```python
from build123d import *

# Parameters (mm, degrees)
ESQUISSE1_R              = 50
BOSS_EXTRU_1_DEPTH       = 22
ESQUISSE5_R              = 6
ENL_V_MAT_EXTRU_6_DEPTH  = 22
ESQUISSE7_R              = 6
ENL_V_MAT_EXTRU_7_DEPTH  = 22
ESQUISSE8_R              = 6
ENL_V_MAT_EXTRU_8_DEPTH  = 22
ESQUISSE9_R              = 6
ENL_V_MAT_EXTRU_9_DEPTH  = 22
ESQUISSE10_R             = 6
ENL_V_MAT_EXTRU_10_DEPTH = 22
ESQUISSE11_R             = 6
ENL_V_MAT_EXTRU_11_DEPTH = 22
ESQUISSE12_R             = 6
ENL_V_MAT_EXTRU_12_DEPTH = 22
ESQUISSE13_R             = 6
ENL_V_MAT_EXTRU_13_DEPTH = 22
ESQUISSE14_R             = 10
ENL_V_MAT_EXTRU_15_DEPTH = 18
ESQUISSE15_R             = 2
ENL_V_MAT_EXTRU_16_DEPTH = 4


with BuildPart() as part:
    # Esquisse1 → Boss.-Extru.1 (new body)
    with BuildSketch(Plane(origin=(0, 0, 0), x_dir=(1, 0, 0), z_dir=(0, 1, 0))):
        with Locations(Location((0, 0, 0), (0, 0, 270))):
            Circle(ESQUISSE1_R)
    extrude(amount=BOSS_EXTRU_1_DEPTH)

    # Esquisse5 → Enlèv. mat.-Extru.6 (cut)
    with BuildSketch(Plane(origin=(0, 0, 0), x_dir=(-1, 0, 0), z_dir=(0, -1, 0))):
        with Locations(Location((-17.68, 17.68, 0), (0, 0, 90))):
            Circle(ESQUISSE5_R)
    extrude(amount=-ENL_V_MAT_EXTRU_6_DEPTH, mode=Mode.SUBTRACT)

    # Esquisse7 → Enlèv. mat.-Extru.7 (cut)
    with BuildSketch(Plane(origin=(0, 0, 0), x_dir=(-1, 0, 0), z_dir=(0, -1, 0))):
        with Locations(Location((18.058126749, -17.68, 0), (0, 0, 90))):
            Circle(ESQUISSE7_R)
    extrude(amount=-ENL_V_MAT_EXTRU_7_DEPTH, mode=Mode.SUBTRACT)

    # Esquisse8 → Enlèv. mat.-Extru.8 (cut)
    with BuildSketch(Plane(origin=(0, 0, 0), x_dir=(-1, 0, 0), z_dir=(0, -1, 0))):
        with Locations(Location((17.68, 17.68, 0), (0, 0, 90))):
            Circle(ESQUISSE8_R)
    extrude(amount=-ENL_V_MAT_EXTRU_8_DEPTH, mode=Mode.SUBTRACT)

    # Esquisse9 → Enlèv. mat.-Extru.9 (cut)
    with BuildSketch(Plane(origin=(0, 0, 0), x_dir=(-1, 0, 0), z_dir=(0, -1, 0))):
        with Locations(Location((-17.68, -17.68, 0), (0, 0, 90))):
            Circle(ESQUISSE9_R)
    extrude(amount=-ENL_V_MAT_EXTRU_9_DEPTH, mode=Mode.SUBTRACT)

    # Esquisse10 → Enlèv. mat.-Extru.10 (cut)
    with BuildSketch(Plane.XZ):
        with Locations(Location((0, 25, 0), (0, 0, 270))):
            Circle(ESQUISSE10_R)
    extrude(amount=-ENL_V_MAT_EXTRU_10_DEPTH, mode=Mode.SUBTRACT)

    # Esquisse11 → Enlèv. mat.-Extru.11 (cut)
    with BuildSketch(Plane(origin=(0, 0, 0), x_dir=(-1, 0, 0), z_dir=(0, -1, 0))):
        with Locations(Location((25, 0, 0), (0, 0, 90))):
            Circle(ESQUISSE11_R)
    extrude(amount=-ENL_V_MAT_EXTRU_11_DEPTH, mode=Mode.SUBTRACT)

    # Esquisse12 → Enlèv. mat.-Extru.12 (cut)
    with BuildSketch(Plane(origin=(0, 0, 0), x_dir=(-1, 0, 0), z_dir=(0, -1, 0))):
        with Locations(Location((-25, 0, 0), (0, 0, 90))):
            Circle(ESQUISSE12_R)
    extrude(amount=-ENL_V_MAT_EXTRU_12_DEPTH, mode=Mode.SUBTRACT)

    # Esquisse13 → Enlèv. mat.-Extru.13 (cut)
    with BuildSketch(Plane(origin=(0, 0, 0), x_dir=(-1, 0, 0), z_dir=(0, -1, 0))):
        with Locations(Location((0, 25, 0), (0, 0, 90))):
            Circle(ESQUISSE13_R)
    extrude(amount=-ENL_V_MAT_EXTRU_13_DEPTH, mode=Mode.SUBTRACT)

    # Esquisse14 → Enlèv. mat.-Extru.15 (cut)
    with BuildSketch(Plane(origin=(0, 0, 0), x_dir=(-1, 0, 0), z_dir=(0, -1, 0))):
        with Locations(Location((0, 0, 0), (0, 0, 90))):
            Circle(ESQUISSE14_R)
    extrude(amount=-ENL_V_MAT_EXTRU_15_DEPTH, mode=Mode.SUBTRACT)

    # Esquisse15 → Enlèv. mat.-Extru.16 (cut)
    with BuildSketch(Plane(origin=(0, 18, 0), x_dir=(-1, 0, 0), z_dir=(0, -1, 0))):
        with Locations(Location((0, 0, 0), (0, 0, 90))):
            Circle(ESQUISSE15_R)
    extrude(amount=-ENL_V_MAT_EXTRU_16_DEPTH, mode=Mode.SUBTRACT)


solid = part.part
```
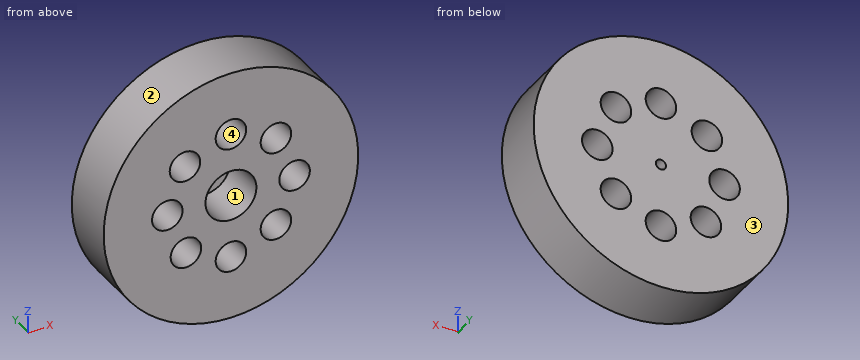
Verification items for the finished model (mm, model axes). Face numbers are marked on the shaded views. Round coordinates to 2 decimals unless told otherwise and drop trailing zeros. Write each loop counter-clockwise with the first axis right and the second up, starting at its lowest first coordinate (ties: lowest second). Pieces come first, ordered by that corner, then holes.
1. Section check D-D on y = 14. State how many separate pieces and enclosed holes the cut face has, plus the area to 3 significant figures.
2. Section check C-C on x = 25. Enter the section's corners in (y, z), plus the area to 3 significant figures.
3. Draft check along Z on the marked faces 1, 2, 3 and 4. Enter one of: +Z half, -Z half, draft (parallel to the pull), parting line (faces both ways), or undercut.
4. Gauge pin test, flat ends, axial feed: P1, Ø1, axis at x = 33.5, y = 10.5, coming from the -Z side; P2, Ø1, axis at x = -38, y = 6, coming from the -Z side; P3, Ø8, axis at x = 17.5, y = 2.5, coming from the +Z side. Record the tip position at first contact, or that the pin passes through.
5. Section check A-A on z = -26.5. Enter the section's corners in (x, y), plus the area to 3 significant figures.
6. Section check B-B on z = 17.68. Enter the section's corners in (x, y), plus the area to 3 significant figures.
7. Scan lines: L1, parallel to X at y = 19.45, z = 0; L2, parallel to Z at x = 23, y = 2.25; L3, parallel to X at y = 15.25, z = 0. Record each from-to range of solid material in increasing order.
Answer:
1. separate pieces: 1
1. enclosed holes: 9
1. area: 6,640 mm2
2. outline: (0, -43.3) - (22, -43.3) - (22, -6) - (0, -6) - close; (0, 6) - (22, 6) - (22, 43.3) - (0, 43.3) - close
2. area: 1,640 mm2
3. face 1: undercut
3. face 2: parting line
3. face 3: draft
3. face 4: undercut
4. P1: stops at z = -37.56
4. P2: stops at z = -33.07
4. P3: stops at z = 48.14
5. outline: (-42.4, 0) - (-5.81, 0) - (-5.81, 22) - (-42.4, 22) - close; (5.81, 0) - (42.4, 0) - (42.4, 22) - (5.81, 22) - close
5. area: 1,610 mm2
6. outline: (-46.77, 0) - (-24.06, 0) - (-24.06, 22) - (-46.77, 22) - close; (-12.06, 0) - (11.68, 0) - (11.68, 22) - (-12.06, 22) - close; (23.68, 0) - (46.77, 0) - (46.77, 22) - (23.68, 22) - close
6. area: 1,530 mm2
7. L1: x = -50 to -31, -19 to -2, 2 to 19, 31 to 50
7. L2: z = -44.4 to -20.45, -14.91 to -5.66, 5.66 to 14.91, 20.45 to 44.4
7. L3: x = -50 to -31, -19 to -10, 10 to 19, 31 to 50
